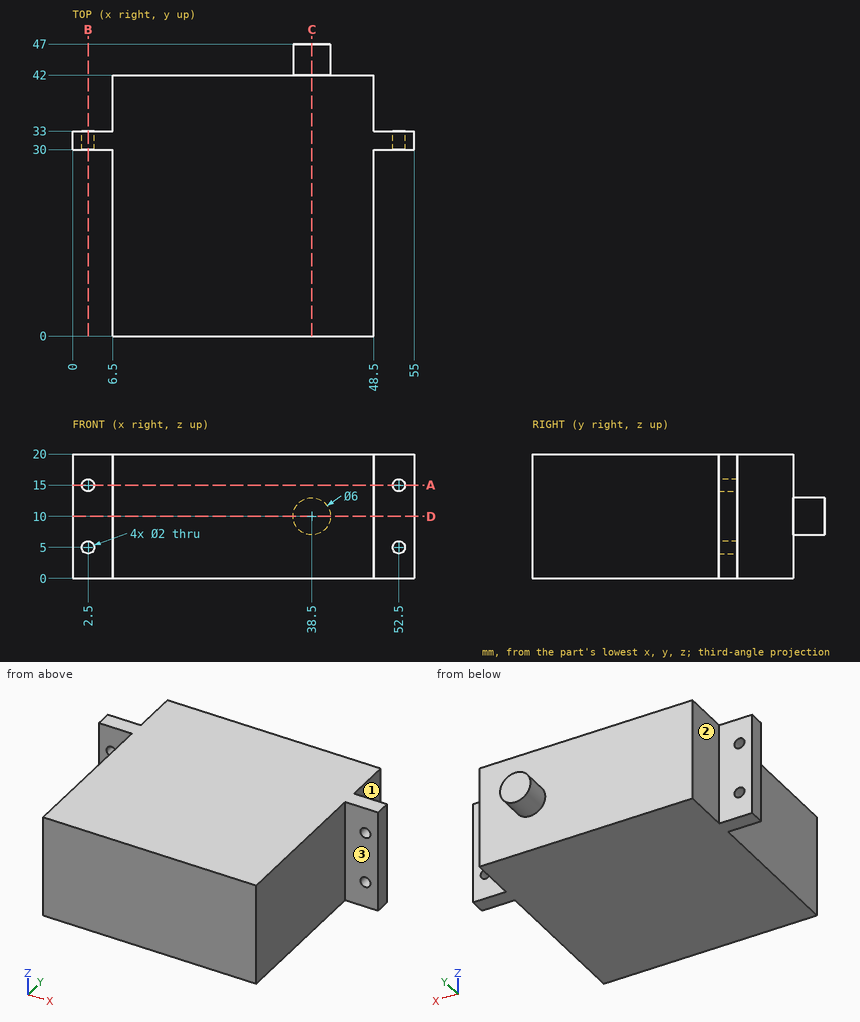
Geometry check sheet. Reference: drawing and pictorial views, mm from the part's lowest x, y, z. A direction names the side the tool comes from. Give positions to 0.01 mm unless a question says otherwise; leave off trailing zeros. Loops run counter-clockwise (first coordinate to the right, second up) from the corner with the lowest first, then second, coordinate; pieces in that order, holes last. Notation, with made-up numbers: (42, 32) -> (54, 32) arc R24 cw to (54, 61) -> close; hole circle Ø3 at (87.25, 65.25). An arc over 180 degrees is marked (long way). Answer in a Markdown table with one row per item. Add a question column.
1) Cross-section at C-C on x = 38.5. Record the boundary of the cut face in (y, z), and give its area (3 significant figures).
2) Cross-section at A-A on z = 15. Record the boundary of the cut face in (x, y).
3) Cross-section at D-D on z = 10. Record the boundary of the cut face in (x, y), and give its area (3 significant figures).
4) Gauge pin test, flat ends, axial feed: P1, Ø2.5, axis at x = 2.5, z = 15, coming from the +Y side; P2, Ø1.5, axis at y = 18, z = 10, coming from the +X side; P3, Ø7, axis at y = 38.5, z = 10.5, coming from the -X side; P4, Ø1.6, axis at x = 2.5, z = 5, coming from the -Y side. Record the tip position at first contact, or that the pin passes through.
5) Material ranges on probe 1 along X at (y, z) = (31.2, 15); probe 2 along Y at (x, z) = (11, 13.5); probe 3 along X at (y, z) = (41, 17), recorded low to high. Write a range as from..to.
6) Cross-section at B-B on x = 2.5. Record the boundary of the cut face in (y, z), and give its area (3 significant figures).
7) Set-up check for the marked faces 1, 2 and 3: record each of +Z, -Z, +X, -X, +Y, -Y from which the full face is reachable in a straight line by a thin tool's end or side.
Outcome:
| question | item | result |
|---|---|---|
| 1 | outline | (0, 0) -> (42, 0) -> (42, 7) -> (47, 7) -> (47, 13) -> (42, 13) -> (42, 20) -> (0, 20) -> close |
| 1 | area | 870 mm^2 |
| 2 | outline | (0, 30) -> (1.5, 30) -> (1.5, 33) -> (0, 33) -> close; (3.5, 30) -> (6.5, 30) -> (6.5, 0) -> (48.5, 0) -> (48.5, 30) -> (51.5, 30) -> (51.5, 33) -> (48.5, 33) -> (48.5, 42) -> (6.5, 42) -> (6.5, 33) -> (3.5, 33) -> close; (53.5, 30) -> (55, 30) -> (55, 33) -> (53.5, 33) -> close |
| 3 | outline | (0, 30) -> (6.5, 30) -> (6.5, 0) -> (48.5, 0) -> (48.5, 30) -> (55, 30) -> (55, 33) -> (48.5, 33) -> (48.5, 42) -> (41.5, 42) -> (41.5, 47) -> (35.5, 47) -> (35.5, 42) -> (6.5, 42) -> (6.5, 33) -> (0, 33) -> close |
| 3 | area | 1,830 mm^2 |
| 4 | P1 | stops at y = 33 |
| 4 | P2 | stops at x = 48.5 |
| 4 | P3 | stops at x = 6.5 |
| 4 | P4 | passes through |
| 5 | probe 1 | x = 0..1.5, 3.5..51.5, 53.5..55 |
| 5 | probe 2 | y = 0..42 |
| 5 | probe 3 | x = 6.5..48.5 |
| 6 | outline | (30, 0) -> (33, 0) -> (33, 4) -> (30, 4) -> close; (30, 6) -> (33, 6) -> (33, 14) -> (30, 14) -> close; (30, 16) -> (33, 16) -> (33, 20) -> (30, 20) -> close |
| 6 | area | 48.0 mm^2 |
| 7 | face 1 | +Z, -Z, +X, +Y |
| 7 | face 2 | +Z, -Z, -X, +Y |
| 7 | face 3 | +Z, -Z, +X, -Y |
